from build123d import *

# Parameters (mm, degrees)
SKETCH2_R               = 2
SKETCH2_R_2             = 1.75
BOSS_EXTRUDE1_DEPTH     = 10
FILLET1_R               = 5
CUT_EXTRUDE1_START      = -15
CUT_EXTRUDE1_DEPTH      = 15
CUT_EXTRUDE2_DEPTH      = 72.414284285
CUT_EXTRUDE2_DEPTH_BACK = 10
SKETCH5_R               = 1.75


with BuildPart() as part:
    # Sketch2 → Boss-Extrude1 (new body)
    with BuildSketch(Plane(origin=(0, 0, 0), x_dir=(1, 0, 0), z_dir=(0, 1, 0))):
        with BuildLine():
            Line((-50, 50), (-28, 50))
            ThreePointArc((-28, 50), (-21.546129824, 42.358449536), (-11.960985068, 39.5))
            Line((-11.960985068, 39.5), (11.960985068, 39.5))
            ThreePointArc((11.960985068, 39.5), (21.546129824, 42.358449536), (28, 50))
            Line((28, 50), (50, 50))
            Line((50, 50), (50, 46))
            Line((50, 46), (36, 46))
            ThreePointArc((36, 46), (30.343145751, 43.656854249), (28, 38))
            Line((28, 38), (28, -38))
            ThreePointArc((28, -38), (30.343145751, -43.656854249), (36, -46))
            Line((36, -46), (50, -46))
            Line((50, -46), (50, -50))
            Line((50, -50), (-50, -50))
            Line((-50, -50), (-50, -46))
            Line((-50, -46), (-36, -46))
            ThreePointArc((-36, -46), (-30.343145751, -43.656854249), (-28, -38))
            Line((-28, -38), (-28, 38))
            ThreePointArc((-28, 38), (-30.343145751, 43.656854249), (-36, 46))
            Line((-36, 46), (-50, 46))
            Line((-50, 46), (-50, 50))
        make_face()
        with Locations(Location((-23.5, 33, 0), (0, 0, 270))):
            Circle(SKETCH2_R, mode=Mode.SUBTRACT)
        with Locations(Location((-23.5, 13, 0), (0, 0, 270))):
            Circle(SKETCH2_R, mode=Mode.SUBTRACT)
        with Locations(Location((23.5, 33, 0), (0, 0, 270))):
            Circle(SKETCH2_R, mode=Mode.SUBTRACT)
        with Locations(Location((23.5, 13, 0), (0, 0, 270))):
            Circle(SKETCH2_R, mode=Mode.SUBTRACT)
        with Locations(Location((-23.5, -33, 0), (0, 0, 270))):
            Circle(SKETCH2_R, mode=Mode.SUBTRACT)
        with Locations(Location((23.5, -33, 0), (0, 0, 270))):
            Circle(SKETCH2_R, mode=Mode.SUBTRACT)
        with Locations(Location((23.5, -13, 0), (0, 0, 270))):
            Circle(SKETCH2_R, mode=Mode.SUBTRACT)
        with Locations(Location((-23.5, -13, 0), (0, 0, 270))):
            Circle(SKETCH2_R, mode=Mode.SUBTRACT)
        with Locations(Location((-20.5, 7.5, 0), (0, 0, 270))):
            Circle(SKETCH2_R_2, mode=Mode.SUBTRACT)
        with Locations(Location((20.5, 7.5, 0), (0, 0, 270))):
            Circle(SKETCH2_R_2, mode=Mode.SUBTRACT)
        with Locations(Location((20.5, -7.5, 0), (0, 0, 270))):
            Circle(SKETCH2_R_2, mode=Mode.SUBTRACT)
        with Locations(Location((-20.5, -7.5, 0), (0, 0, 270))):
            Circle(SKETCH2_R_2, mode=Mode.SUBTRACT)
    extrude(amount=BOSS_EXTRUDE1_DEPTH)

    # Fillet1
    # the kernel refuses this fillet: 5 mm, written as the material it takes off along each edge
    with BuildSketch(Plane(origin=(50, -12.247448714, 50), x_dir=(-1.5667467323505199e-12, 0, -1.0), z_dir=(0, 1, 0)), Plane(origin=(-50, -12.247448714, -50), x_dir=(1.5685230891899197e-12, 0, 1.0), z_dir=(0, 1, 0))) as fillet1_piece_1:
        with BuildLine():
            CenterArc((5, 4.898979486), FILLET1_R, 180, 78.463040967)
            Line((0, 4.898979486), (-0.1, 4.898979486))
            Line((-0.1, 4.898979486), (-0.1, 0))
            Line((-0.1, 0), (0, -0.1))
            ThreePointArc((0, -0.1), (2, -0.1), (3.98, -0.09797959))
            Line((3.98, -0.09797959), (4, 0))
        make_face()
    extrude(amount=34.494897428, mode=Mode.SUBTRACT)
    with BuildSketch(Plane(origin=(-50, -12.247448714, 50), x_dir=(1, 0, 0), z_dir=(0, 1, 0)), Plane(origin=(50, -12.247448714, -50), x_dir=(-1, 0, 0), z_dir=(0, 1, 0))) as fillet1_piece_2:
        with BuildLine():
            CenterArc((4.898979486, 5), FILLET1_R, 191.536959033, 78.463040967)
            Line((0, 4), (-0.09797959, 3.98))
            ThreePointArc((-0.09797959, 3.98), (-0.1, 2), (-0.1, 0))
            Line((-0.1, 0), (0, -0.1))
            Line((0, -0.1), (4.898979486, -0.1))
            Line((4.898979486, -0.1), (4.898979486, 0))
        make_face()
    extrude(amount=34.494897428, mode=Mode.SUBTRACT)

    # Sketch4 → Cut-Extrude1 (cut)
    with BuildSketch(Plane(origin=(0, 10, 0), x_dir=(1, 0, 0), z_dir=(0, 1, 0)).offset(CUT_EXTRUDE1_START)):
        with BuildLine():
            Line((45.101020514, 50), (27.258043608, 48.5))
            ThreePointArc((27.258043608, 48.5), (27.646962091, 49.24112606), (28, 50))
            Line((28, 50), (45.101020514, 50))
        make_face()
        with BuildLine():
            Line((-45.101020514, 50), (-27.258043608, 48.5))
            ThreePointArc((-27.258043608, 48.5), (-27.646962091, 49.24112606), (-28, 50))
            Line((-28, 50), (-45.101020514, 50))
        make_face()
    extrude(amount=CUT_EXTRUDE1_DEPTH, mode=Mode.SUBTRACT)

    # Sketch5 → Cut-Extrude2 (cut, two sides: drawn at the far end of the back side and taken through both)
    with BuildSketch(Plane(origin=(0, 10, 0), x_dir=(1, 0, 0), z_dir=(0, 1, 0)).offset(-CUT_EXTRUDE2_DEPTH_BACK)):
        with Locations(Location((9, -41.531499153, 0), (0, 0, 270))):
            Circle(SKETCH5_R)
        with Locations(Location((-9, -41.531499153, 0), (0, 0, 270))):
            Circle(SKETCH5_R)
        with Locations(Location((5.980492534, 33.6, 0), (0, 0, 270))):
            Circle(SKETCH5_R)
        with Locations(Location((-5.980492534, 33.6, 0), (0, 0, 270))):
            Circle(SKETCH5_R)
    extrude(amount=CUT_EXTRUDE2_DEPTH + CUT_EXTRUDE2_DEPTH_BACK, mode=Mode.SUBTRACT)


solid = part.part
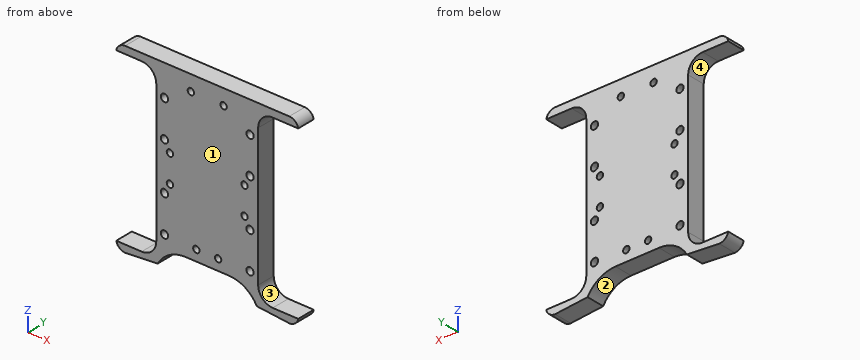
Work out the finished part from the listing and answer in its coordinate system (mm). Face numbers are marked on the shaded views. Round coordinates to 2 decimals unless told otherwise and drop trailing zeros. Loops run counter-clockwise (first coordinate to the right, second up) from the corner with the lowest first, then second, coordinate; pieces in that order, holes last. Notation, with made-up numbers: (-6.75, 45.25) - (7.25, 45.25) arc R21 ccw to (7.25, 69.25) - close; hole circle Ø7 at (36, -0.5). An arc over 180 degrees is marked (long way). One line per item, written item: value.
Q1. Find section A-A on z = 13. Give the vertices of the cut face in (x, y), and give its area (3 significant figures).
Check values:
outline: (-28, 0) - (-25.5, 0) - (-25.5, 10) - (-28, 10) - close; (-21.5, 0) - (21.5, 0) - (21.5, 10) - (-21.5, 10) - close; (25.5, 0) - (28, 0) - (28, 10) - (25.5, 10) - close
area: 480 mm2
Q2. The mould has two halves that part along Z. Classify the marked faces 1, 2, 3 and 4: +Z half, -Z half, draft (parallel to the pull), parting line (faces both ways), or undercut.
Check values:
face 1: draft
face 2: -Z half
face 3: undercut
face 4: undercut
Q3. Find section C-C on z = -33.6. Give the vertices of the cut face in (x, y), and give its area (3 significant figures).
Check values:
outline: (-28, 0) - (-25.41, 0) - (-25.41, 10) - (-28, 10) - close; (-21.59, 0) - (-7.73, 0) - (-7.73, 10) - (-21.59, 10) - close; (-4.23, 0) - (4.23, 0) - (4.23, 10) - (-4.23, 10) - close; (7.73, 0) - (21.59, 0) - (21.59, 10) - (7.73, 10) - close; (25.41, 0) - (28, 0) - (28, 10) - (25.41, 10) - close
area: 414 mm2
Q4. Straight lines are drawn through the part: probe 1 along X at (y, z) = (6.25, 7.5); probe 2 along X at (y, z) = (3.5, 33); probe 3 along X at (y, z) = (7.75, -28.5). For each, find the intervals that lie inside material, in ascending order.
Check values:
probe 1: -28 to -22.25, -18.75 to 18.75, 22.25 to 28
probe 2: -28 to -25.5, -21.5 to 21.5, 25.5 to 28
probe 3: -28 to 28
Q5. Find section D-D on x = 23.5. Give the vertices of the cut face in (y, z), and give its area (3 significant figures).
Check values:
outline: (0, -43.84) - (10, -43.84) - (10, -35) - (0, -35) - close; (0, -31) - (10, -31) - (10, -15) - (0, -15) - close; (0, -11) - (10, -11) - (10, 11) - (0, 11) - close; (0, 15) - (10, 15) - (10, 31) - (0, 31) - close; (0, 35) - (10, 35) - (10, 50) - (0, 50) - close
area: 778 mm2
Q6. Find section B-B on x = 9. Give the vertices of the cut face in (y, z).
Check values:
outline: (0, -39.5) - (10, -39.5) - (10, 39.78) - (0, 39.78) - close; (0, 43.28) - (10, 43.28) - (10, 50) - (0, 50) - close
Q7. Each of these flat-tipped pins is pushed along its axis until it touches: pin 1 Ø5 at (y, z) = (5.5, -21) entering from -X; pin 2 Ø1.5 at (y, z) = (3.5, 19.5) entering from +X; pin 3 Ø2 at (x, z) = (-5.98, -33.6) entering from -Y; pin 4 Ø5 at (x, y) = (3, 4) entering from -Z. Where does it stop, or does it pass through?
Check values:
pin 1: x = -28
pin 2: x = 28
pin 3: through
pin 4: z = -39.5
